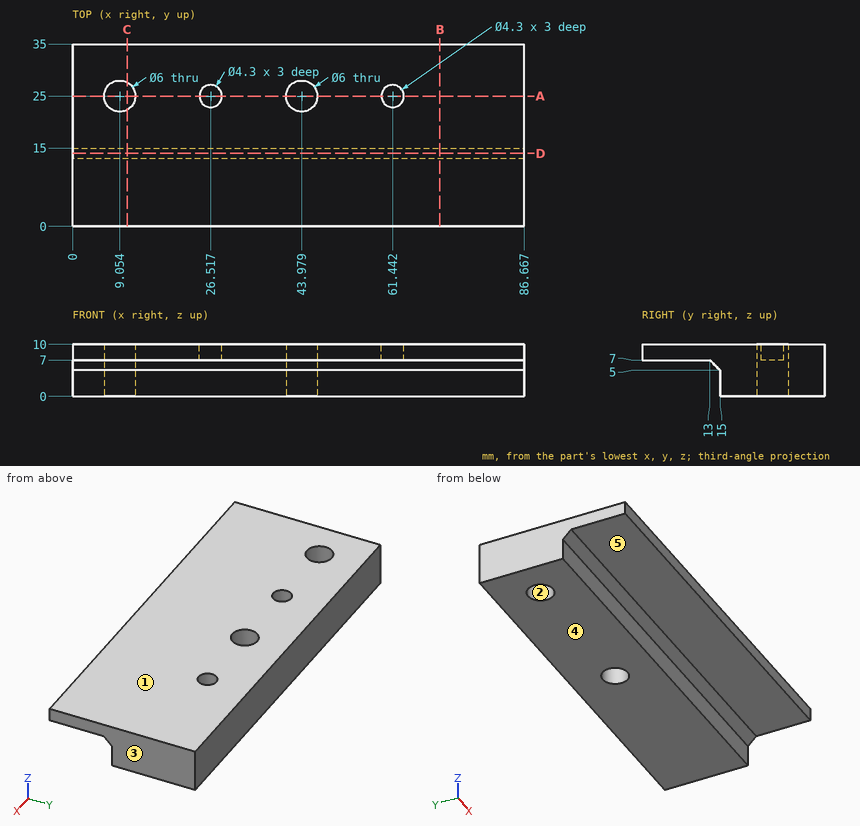
The drawing under review shows one solid part. Ordinate dimensions are in mm from its lowest x, y, z. A direction names the side the tool comes from. Give positions to 0.01 mm unless a question says otherwise; leave off trailing zeros. Write each loop counter-clockwise with the first axis right and the second up, starting at its lowest first coordinate (ties: lowest second). Pieces come first, ordered by that corner, then holes.
1. Tool access review of the marked faces 4 and 5: name each direction out of +Z, -Z, +X, -X, +Y, -Y from which nothing blocks a thin tool from reaching the whole face with its end or side.
2. Add section C-C, the plane x = 10.5. Write out the cut boundary in (y, z), plus the area to 3 significant figures.
3. For P1, Ø3.5, axis at x = 61, y = 26, coming from the +Z side; P2, Ø4, axis at x = 48.5, y = 4, coming from the -Z side; P3, Ø5.5, axis at x = 41, z = 2.5, coming from the -Y side; P4, Ø1.3, axis at x = 26.5, y = 24.5, coming from the +Z side, all flat-tipped, find the tip position at first contact; note any pin that passes through.
4. Add section B-B, the plane x = 70.5. Write out the cut boundary in (y, z).
5. Wall thickness on L1, parallel to X at y = 25, z = 9.05; L2, parallel to X at y = 25, z = 5; L3, parallel to Z at x = 80.5, y = 10.5: over which ranges is each line inside the solid? List them lowest first.
6. Add section A-A, the plane y = 25. Write out the cut boundary in (x, z).
7. Draft analysis for pull direction X (two halves, no side actions). For the marked faces 1, 2 and 3, state which applies: +X half, -X half, draft (parallel to the pull), parting line (faces both ways), or undercut.
8. Add section D-D, the plane y = 14. Write out the cut boundary in (x, z).
Worked answers:
1. face 4: -Z, +X, -X, +Y, -Y
1. face 5: -Z, +X, -X, -Y
2. outline: (0, 7) - (13, 7) - (15, 5) - (15, 0) - (22.37, 0) - (22.37, 10) - (0, 10) - close; (27.63, 0) - (35, 0) - (35, 10) - (27.63, 10) - close
2. area: 194 mm2
3. P1: stops at z = 10
3. P2: stops at z = 7
3. P3: stops at y = 14.75
3. P4: stops at z = 7
4. outline: (0, 7) - (13, 7) - (15, 5) - (15, 0) - (35, 0) - (35, 10) - (0, 10) - close
5. L1: x = 0 to 6.05, 12.05 to 24.37, 28.67 to 40.98, 46.98 to 59.29, 63.59 to 86.67
5. L2: x = 0 to 6.05, 12.05 to 40.98, 46.98 to 86.67
5. L3: z = 7 to 10
6. outline: (0, 0) - (6.05, 0) - (6.05, 10) - (0, 10) - close; (12.05, 0) - (40.98, 0) - (40.98, 10) - (28.67, 10) - (28.67, 7) - (24.37, 7) - (24.37, 10) - (12.05, 10) - close; (46.98, 0) - (86.67, 0) - (86.67, 10) - (63.59, 10) - (63.59, 7) - (59.29, 7) - (59.29, 10) - (46.98, 10) - close
7. face 1: draft
7. face 2: undercut
7. face 3: +X half
8. outline: (0, 6) - (86.67, 6) - (86.67, 10) - (0, 10) - close
